The listing builds one solid part. Answer for the finished solid, in the listing's coordinates (mm). A direction names the side the tool comes from. Give positions to 0.01 mm unless a question says otherwise; leave off trailing zeros. Order: outer loops, then holes, each group sorted by start corner. A loop starts at its lowest first (then second) coordinate and runs counter-clockwise, first axis right, second up. Notation, with made-up numbers: (-11.75, 58) - (17.25, 58) arc R22 cw to (17.25, 77) - close; hole circle Ø6 at (-19, 22). An arc over 180 degrees is marked (long way). Answer as a JSON object with one key per item and string values. Group by question number.
Q1. A cutting plane is placed at A-A, the plane y = 0. Give the vertices of the cut face in (x, z).
Q2. The mould has two halves that part along Y. Classify faces 4 (the face through (0, 0, 1.7)), 5 (the face through (0, 0, -60)), 6 (the face through (-1.5, 0.07, -29.58)): released by +Y, released by -Y, zero draft, split by the parting line, or undercut.
Q3. A cutting plane is placed at B-B, the plane z = -11.5. Give the vertices of the cut face in (x, y), and give its area (3 significant figures).
Q4. Given pin 1 (1 mm diameter, centred on x = 1.5, z = -51.5, fed in from -Y); pin 2 (3 mm diameter, centred on x = 0, y = -0.5, fed in from +Z), each flat-ended and moving along its own axis, determine where each tip first touches the part or whether it passes through.
Q5. A cutting plane is placed at C-C, the plane x = -0.7. Give the vertices of the cut face in (y, z), and give its area (3 significant figures).
Q6. For faces 1 (the face through (1.2, -1.2, 0)), 2 (the face through (0.616, 1.088, 2.359)), 3 (the face through (0.6, 1.3, 3)), determine the directions among +Z, -Z, +X, -X, +Y, -Y from which every point of the face is accessible in a straight line to the end or side of a thin tool.
Q7. Consider line 1 (Z direction, x = -1.6, y = 0.2); line 2 (Z direction, x = 0.65, y = -0.4); line 3 (X direction, y = 0.45, z = -41). Determine where each line is inside the solid, lowest interval first.
Autodesk Inventor part; units mm, degrees
ref_plane "YZ Plane" through (0, 0, 0) normal (1, 0, 0) x (0, 1, 0)
ref_plane "XZ Plane" through (0, 0, 0) normal (0, 1, 0) x (-1, 0, 0)
ref_plane "XY Plane" through (0, 0, 0) normal (0, 0, 1) x (1, 0, 0)
sketch "スケッチ1" plane through (0, 0, 0) normal (0, 0, 1) x (1, 0, 0)
  circle A0 centre (0, 0) radius 1.5
  dimension "d0" = 3
extrude "押し出し1" add sketch "スケッチ1" against normal blind 60
sketch "スケッチ2" plane through (0, 0, 0) normal (0, 0, 1) x (1, 0, 0)
  circle A0 centre (0, 0) radius 2.75
  dimension "d3" = 5.5
extrude "押し出し2" add sketch "スケッチ2" along normal blind 3
sketch "スケッチ3" plane through (0, 0, 3) normal (0, 0, 1) x (1, 0, 0)
  line L0 (0, 1.4434) -> (1.25, 0.7217)
  line L1 (1.25, 0.7217) -> (1.25, -0.7217)
  line L2 (1.25, -0.7217) -> (0, -1.4434)
  line L3 (0, -1.4434) -> (-1.25, -0.7217)
  line L4 (-1.25, -0.7217) -> (-1.25, 0.7217)
  line L5 (-1.25, 0.7217) -> (0, 1.4434)
  point P0 (0, 0)
  point P1 (0, 0)
  dimension "d6" = 2.5
extrude "押し出し3" cut sketch "スケッチ3" against normal blind 1.3
thread "ねじ1"
properties part number "M3キャップボルト 20" material "鋼、高強度、低合金"
Reply:
{
 "1": {"outline": "(-2.75, 0) - (-1.5, 0) - (-1.5, -60) - (1.5, -60) - (1.5, 0) - (2.75, 0) - (2.75, 3) - (1.25, 3) - (1.25, 1.7) - (-1.25, 1.7) - (-1.25, 3) - (-2.75, 3) - close"},
 "2": {"face 4": "undercut", "face 5": "zero draft", "face 6": "split by the parting line"},
 "3": {"outline": "circle Ø3 at (0, 0)", "area": "7.07 mm^2"},
 "4": {"pin 1": "stops at y = -1.12", "pin 2": "stops at z = 3"},
 "5": {"outline": "(-2.66, 0) - (-1.33, 0) - (-1.33, -60) - (1.33, -60) - (1.33, 0) - (2.66, 0) - (2.66, 3) - (1.04, 3) - (1.04, 1.7) - (-1.04, 1.7) - (-1.04, 3) - (-2.66, 3) - close", "area": "172 mm^2"},
 "6": {"face 1": "-Z", "face 2": "+Z", "face 3": "+Z, +X, -X, +Y, -Y"},
 "7": {"line 1": "z = 0 to 3", "line 2": "z = -60 to 1.7", "line 3": "x = -1.43 to 1.43"}
}
